Verification items for the finished model (mm, model axes). A direction names the side the tool comes from. Give positions to 0.01 mm unless a question says otherwise; leave off trailing zeros. Order: outer loops, then holes, each group sorted by start corner. A loop starts at its lowest first (then second) coordinate and runs counter-clockwise, first axis right, second up. Notation, with made-up numbers: (84.5, 28) - (125.5, 28) arc R15 ccw to (125.5, 39) - close; hole circle Ø3 at (0, 18). An arc over 180 degrees is marked (long way). Answer as a JSON object with one key per item and string values. Group by question number.
(1) Section check A-A (y = 2.75). Record the boundary of the cut face in (x, z).
(2) Mould release check, pull along Y, two halves, no side actions. Record for faces 5 (the face through (29, -3.334, 3)), 6 (the face through (-22.004, -10.6, 3.5)), 7 (the face through (12, -12.834, 3)): +Y half, -Y half, draft (parallel to the pull), parting line (faces both ways), or undercut.
(3) Section check B-B (x = -5.5). Record the boundary of the cut face in (y, z), then the cut area to 3 significant figures.
(4) Thickness scan on line 1 (X direction, y = 4, z = 6.75); line 2 (X direction, y = 1.75, z = 6.5); line 3 (Y direction, x = -2, z = 6). Record the ranges inside material, lowest first.
(5) Depth check by flat-ended pin: pin 1 Ø5 at (x, y) = (-7, -9.5) entering from +Z; pin 2 Ø2 at (x, z) = (-7.5, 2.5) entering from -Y; pin 3 Ø1.6 at (y, z) = (-4.5, 4.5) entering from -X; pin 4 Ø1.2 at (y, z) = (-10, 3.5) entering from +X. Enter the tip coordinate at first touch or a pass-through.
(6) Access from +Z, -Z, +X, -X, +Y, -Y to the whole of each face (thin tool, end or side, straight path). Record for faces 1 (the face through (9.32, -12.53, 3.55)), 2 (the face through (-25.035, -10, 3)), 3 (the face through (-26.305, -1.432, 3.451)), 4 (the face through (5, -5.834, 3)).
(7) Section check C-C (x = 13). Record the boundary of the cut face in (y, z).
```python
from build123d import *

# Parameters (mm, degrees)
F1_DEPTH = 7
F2_R     = 1


with BuildPart() as f1:
    # F0 (on Top) → F1 (new body)
    with BuildSketch(Plane.XY):
        with BuildLine():
            Line((-27.834629, -9.334226), (-27.834629, -12.834226))
            Line((-27.834629, -12.834226), (-22.334629, -12.834226))
            Line((-22.334629, -12.834226), (-22.003776, -11.134226))
            Line((-22.003776, -11.134226), (-22.003776, -10.134226))
            Line((-22.003776, -10.134226), (-23.003776, -10.134226))
            Line((-23.003776, -10.134226), (-23.003776, -8.634226))
            Line((-23.003776, -8.634226), (-25.259763, 4.160111))
            ThreePointArc((-25.259763, 4.160111), (-24.651393, 5.028953), (-23.782551, 4.420584))
            Line((-23.782551, 4.420584), (-21.480636, -8.634226))
            Line((-21.480636, -8.634226), (11.996224, -8.634226))
            Line((11.996224, -8.634226), (11.996224, -10.134226))
            Line((11.996224, -10.134226), (9.038184, -10.634226))
            Line((9.038184, -10.634226), (9.038184, -12.834226))
            Line((9.038184, -12.834226), (14.038184, -12.834226))
            Line((14.038184, -12.834226), (18.390972, -8.634226))
            Line((18.390972, -8.634226), (29.887993, -8.634226))
            ThreePointArc((29.887993, -8.634226), (31.816762, -7.835304), (32.615684, -5.906535))
            Line((32.615684, -5.906535), (32.615684, 7.253453))
            ThreePointArc((32.615684, 7.253453), (31.735595, 8.253453), (30.631889, 7.507538))
            Line((30.631889, 7.507538), (28.615684, -0.234227))
            Line((28.615684, -0.234227), (28.615684, -1.234227))
            Line((28.615684, -1.234227), (29.615684, -1.234227))
            Line((29.615684, -1.234227), (29.615684, -3.334226))
            Line((29.615684, -3.334226), (28.115683, -3.334226))
            Line((28.115683, -3.334226), (28.115683, -5.834226))
            Line((28.115683, -5.834226), (18.390972, -5.834226))
            Line((18.390972, -5.834226), (-18.884315, -5.834226))
            Line((-18.884315, -5.834226), (-18.884315, -3.334226))
            Line((-18.884315, -3.334226), (-20.384316, -3.334226))
            Line((-20.384316, -3.334226), (-20.384316, -1.234227))
            Line((-20.384316, -1.234227), (-19.384316, -1.234227))
            Line((-19.384316, -1.234227), (-19.384316, -0.234227))
            Line((-19.384316, -0.234227), (-21.711269, 4.1913))
            Line((-21.711269, 4.1913), (-22.058566, 6.160916))
            ThreePointArc((-22.058566, 6.160916), (-25.111557, 8.41877), (-27.524558, 5.48686))
            Line((-27.524558, 5.48686), (-25.034629, -8.634226))
            Line((-25.034629, -8.634226), (-25.034629, -10.834226))
            ThreePointArc((-25.034629, -10.834226), (-25.684629, -11.484226), (-26.334629, -10.834226))
            Line((-26.334629, -10.834226), (-26.334629, -9.334226))
            Line((-26.334629, -9.334226), (-27.834629, -9.334226))
        make_face()
    extrude(amount=F1_DEPTH)

    # F2
    f2_edges = [f1.edges().sort_by_distance(p)[0] for p in [
        (14.038184, -12.834226, 3.5),
        (-27.834629, -12.834226, 3.5),
        (-22.334629, -12.834226, 3.5),
        (-25.034629, -8.634226, 3.5),
        (18.390972, -8.634226, 3.5),
        (9.038184, -12.834226, 3.5),
        (-21.711269, 4.1913, 3.5),
        (28.615684, -0.234227, 3.5),
        (-19.384316, -0.234227, 3.5),
        (-18.884315, -5.834226, 3.5),
        (-21.480636, -8.634226, 3.5),
        (28.115683, -5.834226, 3.5),
        (-23.003776, -8.634226, 3.5),
        (-27.834629, -9.334226, 3.5),
    ]]
    fillet(f2_edges, radius=F2_R)


solid = f1.part
```
Solutions:
{
 "1": {"outline": "(-27.04, 0) - (-25.01, 0) - (-25.01, 7) - (-27.04, 7) - close; (-23.49, 0) - (-20.95, 0) - (-20.95, 7) - (-23.49, 7) - close; (29.39, 0) - (32.62, 0) - (32.62, 7) - (29.39, 7) - close"},
 "2": {"face 5": "undercut", "face 6": "draft", "face 7": "-Y half"},
 "3": {"outline": "(-8.63, 0) - (-5.83, 0) - (-5.83, 7) - (-8.63, 7) - close", "area": "19.6 mm2"},
 "4": {"line 1": "x = -27.26 to -25.23, -23.71 to -21.61, 29.72 to 32.62", "line 2": "x = -26.87 to -24.83, -23.31 to -20.43, 29.13 to 32.62", "line 3": "y = -8.63 to -5.83"},
 "5": {"pin 1": "stops at z = 7", "pin 2": "stops at y = -8.63", "pin 3": "stops at x = -25.9", "pin 4": "stops at x = 17.6"},
 "6": {"face 1": "+Z, -Z, -Y", "face 2": "+Z, -Z", "face 3": "+Z, -Z, -X", "face 4": "+Z, -Z, +Y"},
 "7": {"outline": "(-12.83, 0) - (-5.83, 0) - (-5.83, 7) - (-12.83, 7) - close"}
}
